Geometry check sheet. Reference: drawing and pictorial views, mm from the part's lowest x, y, z. A direction names the side the tool comes from. Give positions to 0.01 mm unless a question says otherwise; leave off trailing zeros. Order: outer loops, then holes, each group sorted by start corner. A loop starts at its lowest first (then second) coordinate and runs counter-clockwise, first axis right, second up. Notation, with made-up numbers: M 35,61.5 L 45,61.5 A22 cw 45,100.5 Z; hole C -31,36.25 d10. An arc over 180 degrees is marked long. Answer as a JSON object with one key per item and string values. Group by question number.
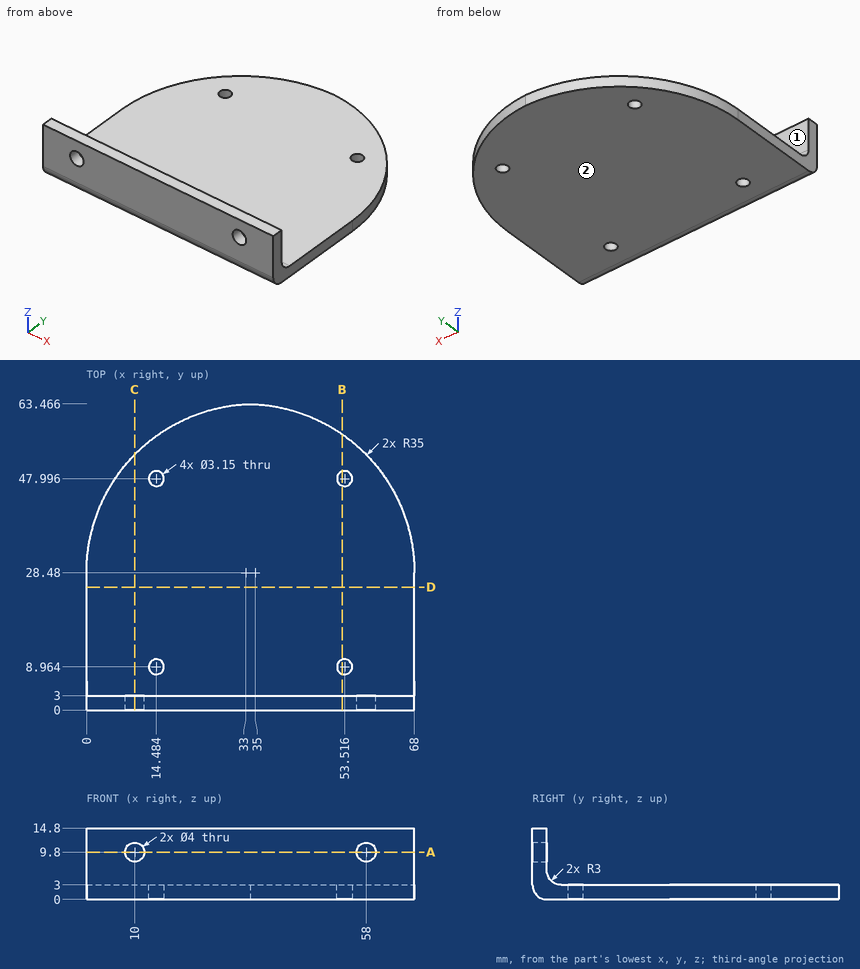
1. Cross-section at B-B (x = 53). Record the cut outline in (y, z), and give its area (3 significant figures).
2. Cross-section at C-C (x = 10). Record the cut outline in (y, z) (1 decimal).
3. Thickness scan on line 1 along X through (y, z) = (1.2, 9.8); line 2 along Y through (x, z) = (36, 5.75); line 3 along Z through (x, y) = (20, 19). Record the ranges inside material, lowest first. Write a range as [from, to].
4. Cross-section at A-A (z = 9.8). Record the cut outline in (x, y), and give its area (3 significant figures).
5. Access from +Z, -Z, +X, -X, +Y, -Y to the whole of each face (thin tool, end or side, straight path). Record for the marked faces 1 and 2.
6. Depth check by flat-ended pin: pin 1 (3 mm diameter, centred on x = 53.52, y = 48, fed in from -Z); pin 2 (4 mm diameter, centred on x = 14.48, y = 48, fed in from +Z); pin 3 (1.5 mm diameter, centred on x = 9.5, z = 5, fed in from +Y). Enter the tip coordinate at first touch or a pass-through.
7. Cross-section at D-D (y = 25.5). Record the cut outline in (x, z).
Report:
{
 "1": {"outline": "M 0,3 A3 ccw 3,0 L 7.48,0 L 7.48,3 L 6,3 A3 cw 3,6 L 3,14.8 L 0,14.8 Z; M 10.45,0 L 46.51,0 L 46.51,3 L 10.45,3 Z; M 49.48,0 L 57.2,0 L 57.2,3 L 49.48,3 Z", "area": "189 mm2"},
 "2": {"outline": "M 0,3 A3 ccw 3,0 L 53,0 L 53,3 L 6,3 A3 cw 3,6 L 3,7.8 L 0,7.8 Z; M 0,11.8 L 3,11.8 L 3,14.8 L 0,14.8 Z"},
 "3": {"line 1": "x = [0, 8], [12, 56], [60, 68]", "line 2": "y = [0, 3.01]", "line 3": "z = [0, 3]"},
 "4": {"outline": "M 0,0 L 8,0 L 8,3 L 0,3 Z; M 12,0 L 56,0 L 56,3 L 12,3 Z; M 60,0 L 68,0 L 68,3 L 60,3 Z", "area": "180 mm2"},
 "5": {"face 1": "+Z, +X, -X, +Y", "face 2": "-Z, +X, -X, +Y, -Y"},
 "6": {"pin 1": "passes through", "pin 2": "stops at z = 3", "pin 3": "stops at y = 3.56"},
 "7": {"outline": "M 0,0 L 68,0 L 68,3 L 0,3 Z"}
}
